Model file for the job. Use its own axes, mm. A direction names the side the tool comes from. Give positions to 0.01 mm unless a question says otherwise; leave off trailing zeros. Write each loop counter-clockwise with the first axis right and the second up, starting at its lowest first coordinate (ties: lowest second). Pieces come first, ordered by that corner, then holes. Notation, with made-up numbers: M 53,57.5 L 110,57.5 A28 ccw 110,90.5 Z; hole C 81.5,-22.5 d8. An arc over 180 degrees is marked long. Answer as a JSON object with one key per item and string values. Group by question number.
```python
from build123d import *

# Parameters (mm, degrees)
AUFSATZ_LINEAR_AUSTRAGEN1_DEPTH      = 20
SCHNITT_LINEAR_AUSTRAGEN1_DEPTH      = 86.117565755
SKIZZE3_R                            = 3.15
SCHNITT_LINEAR_AUSTRAGEN2_DEPTH      = 86.117565755
SCHNITT_LINEAR_AUSTRAGEN3_DEPTH      = 2
SKIZZE5_R                            = 0.75
SCHNITT_LINEAR_AUSTRAGEN4_DEPTH      = 2
SKIZZE6_W                            = 35.5
SKIZZE6_H                            = 6.955295524
AUFSATZ_LINEAR_AUSTRAGEN2_DEPTH      = 20
SKIZZE7_W                            = 7.611739691
SKIZZE7_H                            = 53.192525908
AUFSATZ_LINEAR_AUSTRAGEN3_DEPTH      = 20
SKIZZE8_W                            = 7
SKIZZE8_H                            = 20
AUFSATZ_LINEAR_AUSTRAGEN4_DEPTH      = 27.7
SCHNITT_LINEAR_AUSTRAGEN5_DEPTH      = 26.48
SCHNITT_LINEAR_AUSTRAGEN6_DEPTH      = 6
SCHNITT_LINEAR_AUSTRAGEN6_DEPTH_BACK = 26.48
SKIZZE10_R                           = 1.75
SKIZZE11_R                           = 3
AUFSATZ_LINEAR_AUSTRAGEN5_DEPTH      = 4
SKIZZE12_W                           = 4.692525908
SKIZZE12_H                           = 20
SCHNITT_LINEAR_AUSTRAGEN7_DEPTH      = 131.901413869
SCHNITT_LINEAR_AUSTRAGEN8_DEPTH      = 6.73


with BuildPart() as part:
    # Skizze1 → Aufsatz-Linear austragen1 (new body)
    with BuildSketch(Plane(origin=(0, 0, 0), x_dir=(1, 0, 0), z_dir=(0, 1, 0))):
        with BuildLine():
            Line((0, 59), (0, 0))
            Line((0, 0), (3, 0))
            Line((3, 0), (3, 51.3))
            ThreePointArc((3, 51.3), (4.376598128, 54.623401872), (7.7, 56))
            Line((7.7, 56), (50.3, 56))
            ThreePointArc((50.3, 56), (53.623401872, 54.623401872), (55, 51.3))
            Line((55, 51.3), (55, 0))
            Line((55, 0), (58, 0))
            Line((58, 0), (58, 54.3))
            ThreePointArc((58, 54.3), (56.623401872, 57.623401872), (53.3, 59))
            Line((53.3, 59), (0, 59))
        make_face()
    extrude(amount=AUFSATZ_LINEAR_AUSTRAGEN1_DEPTH)

    # Skizze2 → Schnitt-Linear austragen1 (cut, through all)
    with BuildSketch(Plane(origin=(58, 0, 0), x_dir=(0, 0, -1), z_dir=(1, 0, 0))):
        with BuildLine():
            ThreePointArc((0, 10), (2.928932188, 17.071067812), (10, 20))
            Line((10, 20), (0, 20))
            Line((0, 20), (0, 10))
        make_face()
        with BuildLine():
            ThreePointArc((10, 0), (2.928932188, 2.928932188), (0, 10))
            Line((0, 10), (0, 0))
            Line((0, 0), (10, 0))
        make_face()
    extrude(amount=-SCHNITT_LINEAR_AUSTRAGEN1_DEPTH, mode=Mode.SUBTRACT)

    # Skizze3 → Schnitt-Linear austragen2 (cut, through all)
    with BuildSketch(Plane(origin=(58, 0, 0), x_dir=(0, 0, -1), z_dir=(1, 0, 0))):
        with Locations((10, 10)):
            Circle(SKIZZE3_R)
    extrude(amount=-SCHNITT_LINEAR_AUSTRAGEN2_DEPTH, mode=Mode.SUBTRACT)

    # Skizze4 → Schnitt-Linear austragen3 (cut)
    with BuildSketch(Plane.ZY.offset(-55)):
        with BuildLine():
            Line((-27.5, 7.5), (-12.823894492, 4.145461598))
            ThreePointArc((-12.823894492, 4.145461598), (-3.5, 10), (-12.823894492, 15.854538402))
            Line((-12.823894492, 15.854538402), (-27.5, 12.5))
            ThreePointArc((-27.5, 12.5), (-30, 10), (-27.5, 7.5))
        make_face()
    extrude(amount=-SCHNITT_LINEAR_AUSTRAGEN3_DEPTH, mode=Mode.SUBTRACT)

    # Skizze5 → Schnitt-Linear austragen4 (cut)
    with BuildSketch(Plane.ZY.offset(-57)):
        with Locations((-26.5, 10)):
            Circle(SKIZZE5_R)
        with Locations((-23.5, 10)):
            Circle(SKIZZE5_R)
        with Locations((-20.5, 10)):
            Circle(SKIZZE5_R)
        with Locations((-17.5, 10)):
            Circle(SKIZZE5_R)
    extrude(amount=-SCHNITT_LINEAR_AUSTRAGEN4_DEPTH, mode=Mode.SUBTRACT)

    # Skizze6 → Aufsatz-Linear austragen2 (add)
    with BuildSketch(Plane.XZ):
        with Locations((17.75, -62.477647762)):
            Rectangle(SKIZZE6_W, SKIZZE6_H)
    extrude(amount=-AUFSATZ_LINEAR_AUSTRAGEN2_DEPTH)

    # Skizze7 → Aufsatz-Linear austragen3 (add)
    with BuildSketch(Plane.XZ):
        with Locations((3.805869846, -92.551558478)):
            Rectangle(SKIZZE7_W, SKIZZE7_H)
    extrude(amount=-AUFSATZ_LINEAR_AUSTRAGEN3_DEPTH)

    # Skizze8 → Aufsatz-Linear austragen4 (add)
    with BuildSketch(Plane(origin=(7.611739691, 0, 0), x_dir=(0, 0, -1), z_dir=(1, 0, 0))):
        with Locations((110.955295524, 10)):
            Rectangle(SKIZZE8_W, SKIZZE8_H)
    extrude(amount=AUFSATZ_LINEAR_AUSTRAGEN4_DEPTH)

    # Skizze9 → Schnitt-Linear austragen5 (cut)
    with BuildSketch(Plane(origin=(0, 0, -119.147821432), x_dir=(-1, 0, 0), z_dir=(0, 0, -1))):
        with BuildLine():
            Line((-9.3, 13.5), (-29.794038703, 13.5))
            ThreePointArc((-29.794038703, 13.5), (-31.066830909, 12.972792206), (-31.594038703, 11.7))
            Line((-31.594038703, 11.7), (-31.594038703, 8.3))
            ThreePointArc((-31.594038703, 8.3), (-31.066830909, 7.027207794), (-29.794038703, 6.5))
            Line((-29.794038703, 6.5), (-9.3, 6.5))
            ThreePointArc((-9.3, 6.5), (-8.027207794, 7.027207794), (-7.5, 8.3))
            Line((-7.5, 8.3), (-7.5, 11.7))
            ThreePointArc((-7.5, 11.7), (-8.027207794, 12.972792206), (-9.3, 13.5))
        make_face()
    extrude(amount=-SCHNITT_LINEAR_AUSTRAGEN5_DEPTH, mode=Mode.SUBTRACT)

    # Skizze10 → Schnitt-Linear austragen6 (cut, two sides: drawn at the far end of the back side and taken through both)
    with BuildSketch(Plane(origin=(35.311739691, 0, 0), x_dir=(0, 0, -1), z_dir=(1, 0, 0)).offset(-SCHNITT_LINEAR_AUSTRAGEN6_DEPTH_BACK)):
        with Locations((62.055295524, 15)):
            Circle(SKIZZE10_R)
        with Locations((62.055295524, 5)):
            Circle(SKIZZE10_R)
        with Locations(Location((110.855295524, 5, 0), (0, 0, 180))):
            Circle(SKIZZE10_R)
        with Locations(Location((110.855295524, 15, 0), (0, 0, 180))):
            Circle(SKIZZE10_R)
    extrude(amount=SCHNITT_LINEAR_AUSTRAGEN6_DEPTH + SCHNITT_LINEAR_AUSTRAGEN6_DEPTH_BACK, mode=Mode.SUBTRACT)

    # Skizze11 → Aufsatz-Linear austragen5 (add)
    with BuildSketch(Plane.ZY):
        with Locations((-96.955295524, 10)):
            Circle(SKIZZE11_R)
    extrude(amount=AUFSATZ_LINEAR_AUSTRAGEN5_DEPTH)

    # Skizze12 → Schnitt-Linear austragen7 (cut, through all)
    with BuildSketch(Plane(origin=(7.611739691, 0, 0), x_dir=(0, 0, -1), z_dir=(1, 0, 0))):
        with Locations((116.801558478, 10)):
            Rectangle(SKIZZE12_W, SKIZZE12_H)
    extrude(amount=-SCHNITT_LINEAR_AUSTRAGEN7_DEPTH, mode=Mode.SUBTRACT)

    # Skizze13 → Schnitt-Linear austragen8 (cut)
    with BuildSketch(Plane.ZY):
        with BuildLine():
            Line((-47.3, 3), (-31.3, 3))
            ThreePointArc((-31.3, 3), (-29.885786438, 3.585786438), (-29.3, 5))
            Line((-29.3, 5), (-29.3, 15))
            ThreePointArc((-29.3, 15), (-29.885786438, 16.414213562), (-31.3, 17))
            Line((-31.3, 17), (-47.3, 17))
            ThreePointArc((-47.3, 17), (-48.714213562, 16.414213562), (-49.3, 15))
            Line((-49.3, 15), (-49.3, 5))
            ThreePointArc((-49.3, 5), (-48.714213562, 3.585786438), (-47.3, 3))
        make_face()
    extrude(amount=-SCHNITT_LINEAR_AUSTRAGEN8_DEPTH, mode=Mode.SUBTRACT)


solid = part.part
```
Q1. Drop flat-ended pins along their axis: P1, Ø3.5, axis at y = 14.5, z = -111, coming from the +X side; P2, Ø7.5, axis at y = 12, z = -63, coming from the +X side; P3, Ø3.5, axis at y = 9, z = -110, coming from the -X side. Give the stop position or say it passes through.
Q2. Slice it at C-C, the plane y = 18.5. Write the cut outline in (x, z), then the cut area to 3 significant figures.
Q3. Slice it at B-B, the plane z = -11.5. Write the cut outline in (x, y).
Q4. Two-plate mould, pull along Y, no slides. Class faces 1 (the cylindrical face through (-1.972, 10.901, -94.094)), 2 (the flat face through (8.832, 5, -111)), 3 (the flat face through (-4, 10, -97)): +Y half, -Y half, draft (parallel to the pull), parting line (faces both ways), or undercut.
Q5. 3-axis set-ups, long thin cutter, end or side, ignore diameter. For faces 4 (the flat face through (45, 10, -59)), 5 (the cylindrical face through (53.587, 9.86, -54.66)), 6 (the flat face through (21, 10, -65.955)), 7 (the cylindrical face through (55.986, 9.816, -3.503)), 8 (the flat face through (20, 6.5, -109)): which of +Z, -Z, +X, -X, +Y, -Y reach the whole face in a straight line?
Q6. Wall check: L1, parallel to Z at x = 25.5, y = 5; L2, parallel to X at y = 13.75, z = -26.5; L3, parallel to Y at x = 57.7, z = -20.5. Give the ranges that are in metal, low to high.
Q7. Slice it at D-D, the plane z = -78.5. Write the cut outline in (x, y), then the cut area to 3 significant figures.
Q8. Slice it at A-A, the plane x = 11.5. Write the cut outline in (y, z).
Solved:
{
 "1": {"P1": "stops at x = 35.31", "P2": "stops at x = 35.5", "P3": "stops at x = 0"},
 "2": {"outline": "M 0,-114.46 L 35.31,-114.46 L 35.31,-107.46 L 7.61,-107.46 L 7.61,-65.96 L 35.5,-65.96 L 35.5,-59 L 53.3,-59 A4.7 ccw 58,-54.3 L 58,-4.73 L 55,-4.73 L 55,-51.3 A4.7 cw 50.3,-56 L 7.7,-56 A4.7 cw 3,-51.3 L 3,-4.73 L 0,-4.73 Z", "area": "1,300 mm²"},
 "3": {"outline": "M 0,0 L 3,0 L 3,7.23 L 0,7.23 Z; M 0,12.77 L 3,12.77 L 3,20 L 0,20 Z; M 55,0 L 58,0 L 58,7.23 L 57,7.23 L 57,3.68 L 55,3.68 Z; M 55,16.32 L 57,16.32 L 57,12.77 L 58,12.77 L 58,20 L 55,20 Z"},
 "4": {"face 1": "parting line", "face 2": "undercut", "face 3": "draft"},
 "5": {"face 4": "-Z, +X, +Y, -Y", "face 5": "+Z, +Y, -Y", "face 6": "+X, +Y, -Y", "face 7": "none", "face 8": "-Z"},
 "6": {"L1": "z = -114.46 to -112.61, -109.11 to -107.46, -65.96 to -63.81, -60.31 to -56", "L2": "x = 0 to 3, 55 to 58", "L3": "y = 0 to 9.25, 10.75 to 20"},
 "7": {"outline": "M 0,0 L 7.61,0 L 7.61,20 L 0,20 Z", "area": "152 mm²"},
 "8": {"outline": "M 0,-114.46 L 6.5,-114.46 L 6.5,-111.76 A1.75 cw long 6.5,-109.95 L 6.5,-107.46 L 0,-107.46 Z; M 0,-65.96 L 20,-65.96 L 20,-56 L 0,-56 Z; M 13.5,-114.46 L 20,-114.46 L 20,-107.46 L 13.5,-107.46 L 13.5,-109.95 A1.75 cw long 13.5,-111.76 Z; hole C 5,-62.06 d3.5; hole C 15,-62.06 d3.5"}
}
